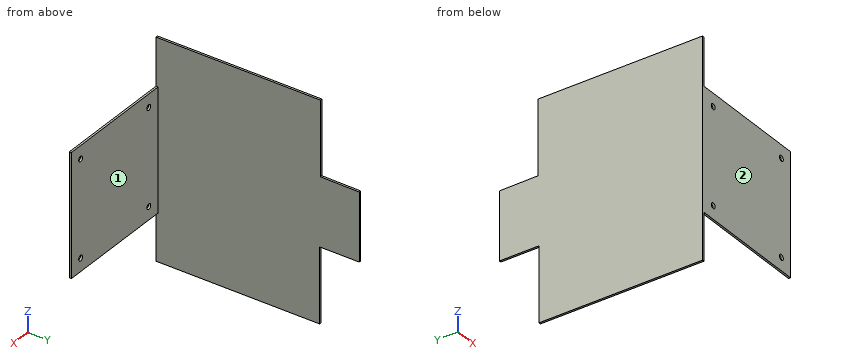
```python
from build123d import *

# Parameters (mm, degrees)
SKETCH1_W           = 320
SKETCH1_H           = 300
BOSS_EXTRUDE1_DEPTH = 3
SKETCH2_W           = 180
SKETCH2_H           = 180
SKETCH2_R           = 4
BOSS_EXTRUDE2_DEPTH = 3
CUT_EXTRUDE1_DEPTH  = 10


with BuildPart() as part:
    # Sketch1 → Boss-Extrude1 (new body)
    with BuildSketch(Plane(origin=(0, 0, 0), x_dir=(0, 0, -1), z_dir=(1, 0, 0))):
        Rectangle(SKETCH1_W, SKETCH1_H)
    extrude(amount=BOSS_EXTRUDE1_DEPTH)

    # Sketch2 → Boss-Extrude2 (add)
    with BuildSketch(Plane.XZ.offset(150)):
        with Locations((93, 0)):
            Rectangle(SKETCH2_W, SKETCH2_H)
        with Locations((22.29, -70.71)):
            Circle(SKETCH2_R, mode=Mode.SUBTRACT)
        with Locations((22.29, 70.71)):
            Circle(SKETCH2_R, mode=Mode.SUBTRACT)
        with Locations((163.71, 70.71)):
            Circle(SKETCH2_R, mode=Mode.SUBTRACT)
        with Locations((163.71, -70.71)):
            Circle(SKETCH2_R, mode=Mode.SUBTRACT)
    extrude(amount=-BOSS_EXTRUDE2_DEPTH)

    # Sketch3 → Cut-Extrude1 (cut)
    with BuildSketch(Plane(origin=(3, 0, 0), x_dir=(0, 0, -1), z_dir=(1, 0, 0))):
        Polygon((-50, 152), (-50.5, 92.5), (-174.995322546, 92.5), (-174.995322546, 153.849759006), (-150, 158.899747984), align=None)
        Polygon((186.01679007, 162.206902793), (50, 152), (50, 91.655462185), (186.01679007, 91.655462185), align=None)
    extrude(amount=-CUT_EXTRUDE1_DEPTH, mode=Mode.SUBTRACT)


solid = part.part
```
Input: part model. Units: mm. Frame: model coordinates. Face numbers are marked on the shaded views. A direction names the side the tool comes from. Coordinates: 2 decimals unless noted, no trailing zeros. Write each loop counter-clockwise with the first axis right and the second up, starting at its lowest first coordinate (ties: lowest second). Pieces come first, ordered by that corner, then holes. Notation, with made-up numbers: (4, 65) -> (12, 65) arc R20 cw to (12, 76) -> close; hole circle Ø5 at (-3, 53.5). An arc over 180 degrees is marked (long way). Write each question's results on one line, items separated by ' | '.
Item 1: Set-up query: the marked faces 1 and 2. Return all of +Z, -Z, +X, -X, +Y, -Y with unobstructed straight access to the full face (end or side cutting, diameter ignored); none if empty.
Conclusion:
face 1: +Z, -Z, +X, +Y | face 2: +Z, -Z, +X, -X, -Y
Item 2: Section query A-A on x = 22.29. Return loops of the section in (y, z).
Conclusion:
outline: (-150, -90) -> (-147, -90) -> (-147, -74.71) -> (-150, -74.71) -> close; (-150, -66.71) -> (-147, -66.71) -> (-147, 66.71) -> (-150, 66.71) -> close; (-150, 74.71) -> (-147, 74.71) -> (-147, 90) -> (-150, 90) -> close
Item 3: Section query B-B on z = 70.71. Return loops of the section in (x, y), plus the area to 3 significant figures.
Conclusion:
outline: (0, -150) -> (18.29, -150) -> (18.29, -147) -> (3, -147) -> (3, 92.5) -> (0, 92.5) -> close; (26.29, -150) -> (159.71, -150) -> (159.71, -147) -> (26.29, -147) -> close; (167.71, -150) -> (183, -150) -> (183, -147) -> (167.71, -147) -> close | area: 1,220 mm^2
Item 4: Section query D-D on y = -29. Return loops of the section in (x, z).
Conclusion:
outline: (0, -160) -> (3, -160) -> (3, 160) -> (0, 160) -> close
Item 5: Section query C-C on z = 32. Return loops of the section in (x, y), plus the area to 3 significant figures.
Conclusion:
outline: (0, -150) -> (183, -150) -> (183, -147) -> (3, -147) -> (3, 150) -> (0, 150) -> close | area: 1,440 mm^2
Item 6: Material intervals for probe 1 along Z at (x, y) = (22.29, -147.95); probe 2 along X at (y, z) = (-38, -83.5); probe 3 along Y at (x, z) = (123.5, 78), sorted ascending.
Conclusion:
probe 1: z = -90 to -74.71, -66.71 to 66.71, 74.71 to 90 | probe 2: x = 0 to 3 | probe 3: y = -150 to -147
Item 7: Pin query (flat end, axial travel): pin 1 Ø0.9 at (x, y) = (2, 114.5) entering from -Z; pin 2 Ø3.5 at (x, y) = (115, -148) entering from +Z; pin 3 Ø12 at (y, z) = (-105, -32) entering from +X; pin 4 Ø7 at (x, z) = (22.29, 70.71) entering from -Y. Return the tip coordinate at first contact, or that it passes through.
Conclusion:
pin 1: stops at z = -50 | pin 2: stops at z = 90 | pin 3: stops at x = 3 | pin 4: passes through
